CAD build for the part. Positions are in the model's coordinates, mm. Face numbers are marked on the shaded views. A direction names the side the tool comes from. Coordinates: 2 decimals unless noted, no trailing zeros. Loops run counter-clockwise (first coordinate to the right, second up) from the corner with the lowest first, then second, coordinate; pieces in that order, holes last. Notation, with made-up numbers: (55, -37) - (72, -37) arc R22 cw to (72, -25) - close; hole circle Ø6 at (70, 2.5). An arc over 180 degrees is marked (long way). Put each result on its own line as item: value.
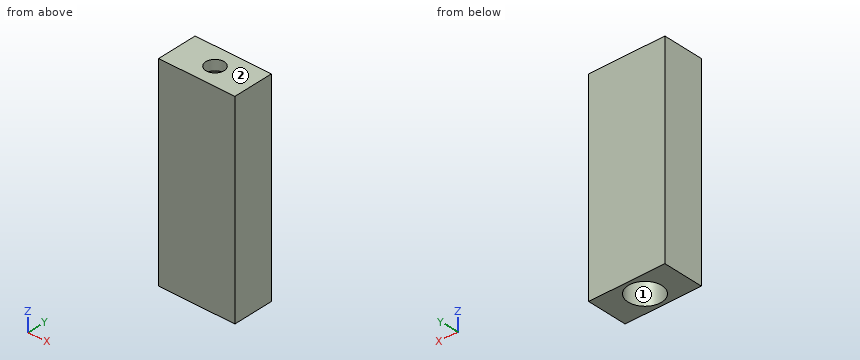
```python
from build123d import *

# Parameters (mm, degrees)
CYLINDER044_R     = 3.3
CYLINDER044_DEPTH = 35
CYLINDER043_R     = 1.8
CYLINDER043_DEPTH = 40
BOX022_W          = 15
BOX022_H          = 8
BOX022_DEPTH      = 40


with BuildPart() as cone001:
    # Cone001 → Cone001 (revolve)
    with BuildSketch(Plane(origin=(7.5, 4, 35), x_dir=(1, 0, 0), z_dir=(0, -1, 0))):
        Polygon((0, 0), (3.3, 0), (1.8, 3), (0, 3), align=None)
    revolve(axis=Axis((7.5, 4, 35), (0, 0, 1)))


with BuildPart() as cylinder009:
    # Cylinder044 → Cylinder044 (new body)
    with BuildSketch(Plane(origin=(7.5, 4, 0), x_dir=(1, 0, 0), z_dir=(0, 0, 1))):
        Circle(CYLINDER044_R)
    extrude(amount=CYLINDER044_DEPTH)


with BuildPart() as fusion016:
    # Cylinder043 → Cylinder043 (new body)
    with BuildSketch(Plane(origin=(7.5, 4, 0), x_dir=(1, 0, 0), z_dir=(0, 0, 1))):
        Circle(CYLINDER043_R)
    extrude(amount=CYLINDER043_DEPTH)

    # Fusion016: union Cone001, Cylinder009
    add(cone001.part)
    add(cylinder009.part)


with BuildPart() as top_stop_trigger_cut:
    # Box022 → Box022 (new body)
    with BuildSketch(Plane.XY):
        with Locations((7.5, 4)):
            Rectangle(BOX022_W, BOX022_H)
    extrude(amount=BOX022_DEPTH)

    # Cut016: cut Fusion016
    add(fusion016.part, mode=Mode.SUBTRACT)


solid = top_stop_trigger_cut.part
```
Q1. Slice it at A-A, the plane x = 7.5. Give the cut face in (y, z).
Determined:
outline: (0, 0) - (0.7, 0) - (0.7, 35) - (2.2, 38) - (2.2, 40) - (0, 40) - close; (5.8, 38) - (7.3, 35) - (7.3, 0) - (8, 0) - (8, 40) - (5.8, 40) - close
Q2. Tool access for the marked faces 1 and 2: list every direction of +Z, -Z, +X, -X, +Y, -Y with a clear straight run to the whole face (end or side of a thin tool).
Determined:
face 1: -Z
face 2: +Z, +X, -X, +Y, -Y
Q3. Wall check: L1, parallel to Y at x = 7.5, z = 14; L2, parallel to X at y = 3.75, z = 19; L3, parallel to Y at x = 8.75, z = 23.5. Give the ranges that are in metal, low to high. Write a range as from..to.
Determined:
L1: 0..0.7, 7.3..8
L2: 0..4.21, 10.79..15
L3: 0..0.95, 7.05..8
Q4. Slice it at B-B, the plane z = 13. Give the cut face in (x, y), then the cut area to 3 significant figures.
Determined:
outline: (0, 0) - (15, 0) - (15, 8) - (0, 8) - close; hole circle Ø6.6 at (7.5, 4)
area: 85.8 mm2
Q5. Slice it at C-C, the plane y = 4. Give the cut face in (x, z).
Determined:
outline: (0, 0) - (4.2, 0) - (4.2, 35) - (5.7, 38) - (5.7, 40) - (0, 40) - close; (9.3, 38) - (10.8, 35) - (10.8, 0) - (15, 0) - (15, 40) - (9.3, 40) - close
Q6. Pin check, flat tips, straight feed: pin 1 Ø2 at (y, z) = (3, 19.5) entering from -X; pin 2 Ø2 at (x, y) = (7.5, 4) entering from -Z. Stop position of each tip, or through.
Determined:
pin 1: x = 0
pin 2: through
